The listing builds one solid part. Answer for the finished solid, in the listing's coordinates (mm). A direction names the side the tool comes from. Round coordinates to 2 decimals unless told otherwise and drop trailing zeros. Write each loop counter-clockwise with the first axis right and the second up, starting at its lowest first coordinate (ties: lowest second). Pieces come first, ordered by that corner, then holes. Notation, with made-up numbers: (-22, 18.5) - (-14, 18.5) arc R26 cw to (-14, 39.5) - close; hole circle Ø6 at (28, 2). An arc over 180 degrees is marked (long way). Use a Markdown table: item, result. Add a question column.
1) A cutting plane is placed at C-C (z = 0.55). State how many separate pieces and enclosed holes the cut face has, then the cut area to 3 significant figures.
2) A cutting plane is placed at D-D (x = 85.5). Give the vertices of the cut face in (y, z).
3) A cutting plane is placed at B-B (y = 48.5). Give the vertices of the cut face in (x, z), then the cut area to 3 significant figures.
4) A tool of negligible diameter and unlimited length cuts with its end or side. For faces 1 (the cylindrical face through (96.36, 73.78, 1.63)), 2 (the flat face through (113, 90.8, 1.6)), from which of +Z, -Z, +X, -X, +Y, -Y can it reach the whole face along a straight path? Write none if from no direction.
5) Find the intervals of material crossed by probe 1 along X at (y, z) = (48.5, 1.65); probe 2 along Y at (x, z) = (65, 1.1); probe 3 along X at (y, z) = (80.5, 1.2), in increasing order. Write a range as from..to.
6) A cutting plane is placed at A-A (x = 59). Give the vertices of the cut face in (y, z).
7) Determine the mould class of faces 3 (the cylindrical face through (102.313, 46.888, 1.628)), 4 (the cylindrical face through (55.615, 31.343, 1.628)), 5 (the flat face through (58, 29, 3.302)), 6 (the flat face through (4.766, 91.18, 1.628)) for opening direction X: +X half, -X half, draft (parallel to the pull), parting line (faces both ways), or undercut.
8) This flat-tipped pin is pushed along its axis until it touches: P1, Ø4.5, axis at x = 64.39, y = 88.41, coming from the +Z side. Where does it stop, or does it pass through?
```python
from build123d import *

# Parameters (mm, degrees)
SKETCH1_R      = 14.280154621
SKETCH1_R_2    = 3.175
SKETCH1_R_3    = 2.445943814
EXTRUDE1_DEPTH = 3.302


with BuildPart() as part:
    # Sketch1 → Extrude1 (new body)
    with BuildSketch(Plane.XY):
        Polygon((122.018241697, 78.932176277), (103.665120274, 103.090232189), (13.814462921, 103.090232189), (-4.538658503, 78.932176277), (-4.538658503, -19.747260734), (122.018241697, -19.747260734), align=None)
        with Locations((58.710249945, 45.283910371)):
            Circle(SKETCH1_R, mode=Mode.SUBTRACT)
        with Locations((108.031447678, 83.274598732)):
            Circle(SKETCH1_R_2, mode=Mode.SUBTRACT)
        with Locations((64.386022104, 88.408658993)):
            Circle(SKETCH1_R_3, mode=Mode.SUBTRACT)
        with Locations(Location((101.914361119, 39.6877037, 0), (0, 0, 180))):
            Circle(SKETCH1_R_3, mode=Mode.SUBTRACT)
        with BuildLine():
            ThreePointArc((105.584923307, 50.978901238), (96.144059082, 74.065464486), (76.258457488, 89.121432379))
            ThreePointArc((76.258457488, 89.121432379), (71.3691103, 86.793097674), (74.070723534, 82.099682674))
            ThreePointArc((74.070723534, 82.099682674), (90.512346787, 69.36651562), (98.311501424, 50.088712183))
            ThreePointArc((98.311501424, 50.088712183), (102.393306893, 46.897095769), (105.584923307, 50.978901238))
        make_face(mode=Mode.SUBTRACT)
    extrude(amount=EXTRUDE1_DEPTH)


solid = part.part
```
Entries:
| question | item | result |
|---|---|---|
| 1 | separate pieces | 1 |
| 1 | enclosed holes | 5 |
| 1 | area | 14,000 mm² |
| 2 | outline | (-19.75, 0) - (74.84, 0) - (74.84, 3.3) - (-19.75, 3.3) - close; (84.17, 0) - (103.09, 0) - (103.09, 3.3) - (84.17, 3.3) - close |
| 3 | outline | (-4.54, 0) - (44.8, 0) - (44.8, 3.3) - (-4.54, 3.3) - close; (72.62, 0) - (98.9, 0) - (98.9, 3.3) - (72.62, 3.3) - close; (105, 0) - (122.02, 0) - (122.02, 3.3) - (105, 3.3) - close |
| 3 | area | 306 mm² |
| 4 | face 1 | +Z, -Z |
| 4 | face 2 | +Z, -Z, +X, +Y |
| 5 | probe 1 | x = -4.54..44.8, 72.62..98.9, 105..122.02 |
| 5 | probe 2 | y = -19.75..32.46, 58.1..86.04, 90.78..103.09 |
| 5 | probe 3 | x = -3.35..77.45, 90.17..106.49, 109.57..120.83 |
| 6 | outline | (-19.75, 0) - (31.01, 0) - (31.01, 3.3) - (-19.75, 3.3) - close; (59.56, 0) - (103.09, 0) - (103.09, 3.3) - (59.56, 3.3) - close |
| 7 | face 3 | undercut |
| 7 | face 4 | undercut |
| 7 | face 5 | draft |
| 7 | face 6 | -X half |
| 8 | P1 | passes through |
